For this review, take the finished solid that the model builds, in its own axes (mm). A direction names the side the tool comes from. Coordinates: 2 decimals unless noted, no trailing zeros. Loops run counter-clockwise (first coordinate to the right, second up) from the corner with the lowest first, then second, coordinate; pieces in that order, holes last. Notation, with made-up numbers: M 15,67 L 65,67 A26 ccw 65,85 Z; hole C 69.25,-18 d8. An arc over 180 degrees is marked long. Answer as a JSON object with one key per item and string values. Group by question number.
Item 1: Add section B-B (z = -44). State the section outline as (x, y) points, then the cut area to 3 significant figures.
Item 2: Add section D-D (y = 3.5). State the section outline as (x, z) points.
Item 3: Add section A-A (y = 22). State the section outline as (x, z) points, then the cut area to 3 significant figures.
Item 4: Insertion check: pin 1 (6 mm diameter, centred on x = -32, y = 5.5, fed in from -Z); pin 2 (6 mm diameter, centred on x = -5.5, z = -49.5, fed in from +Y); pin 3 (5 mm diameter, centred on x = -46.5, y = 19.5, fed in from -Z). Each pin has a flat end and moves straight along its axis. Give the tip position at first contact, or say it passes through.
Item 5: Wall thickness on L1, parallel to Z at x = -88.5, y = 27; L2, parallel to Y at x = 7, z = -45; L3, parallel to X at y = 8, z = -52: over which ranges is each line inside the solid? List them lowest first. Write a range as from..to.
Item 6: Tool access review of faces 5 (the face through (-41, 23, -42.5)), 6 (the face through (7, 2.5, -49)), 7 (the face through (-41, 30.911, -37)): name each direction out of +Z, -Z, +X, -X, +Y, -Y from which nothing blocks a thin tool from reaching the whole face with its end or side.
Item 7: Mouldability with a two-part tool opening along Z and no side actions: class faces 1 (the face through (-81, 15, -47)), 2 (the face through (-41, 16, -32.5)), 3 (the face through (7.057, 8.838, -51.855)), 4 (the face through (-40.9, 7.4, -42.5)) as +Z half, -Z half, draft (parallel to the pull), parting line (faces both ways), or undercut.
Item 8: Add section C-C (x = -61.5). State the section outline as (y, z) points, then the cut area to 3 significant figures.
from build123d import *

# Parameters (mm, degrees)
BOSS_EXTRUDE1_DEPTH = 15
SKETCH5_W           = 107
SKETCH5_H           = 15.91087052
BOSS_EXTRUDE2_DEPTH = 10
CUT_EXTRUDE1_START  = -15
SKETCH6_R           = 2.9
CUT_EXTRUDE1_DEPTH  = 12.5
SKETCH7_R           = 2.9
CUT_EXTRUDE2_DEPTH  = 12.5


with BuildPart() as part:
    # Sketch4 → Boss-Extrude1 (new body)
    with BuildSketch(Plane(origin=(0, 0, 0), x_dir=(1, 0, 0), z_dir=(0, 1, 0))):
        with BuildLine():
            Line((13.184906132, 32.500351338), (-93.815093868, 32.500351338))
            Line((-93.815093868, 32.500351338), (-93.815093868, 48.957491145))
            ThreePointArc((-93.815093868, 48.957491145), (-87.815093868, 54.957491145), (-81.815093868, 48.957491145))
            ThreePointArc((-81.815093868, 48.957491145), (-40.315093868, 42.500341518), (1.184906132, 48.957491145))
            ThreePointArc((1.184906132, 48.957491145), (7.184906132, 54.957491145), (13.184906132, 48.957491145))
            Line((13.184906132, 48.957491145), (13.184906132, 32.500351338))
        make_face()
    extrude(amount=BOSS_EXTRUDE1_DEPTH)

    # Sketch5 → Boss-Extrude2 (add)
    with BuildSketch(Plane.XY.offset(-32.500351338)):
        with Locations((-40.315093868, 22.95543526)):
            Rectangle(SKETCH5_W, SKETCH5_H)
    extrude(amount=-BOSS_EXTRUDE2_DEPTH)

    # Sketch6 → Cut-Extrude1 (cut)
    with BuildSketch(Plane.XZ.offset(CUT_EXTRUDE1_START)):
        with Locations(Location((7.184906132, -48.957491145, 0), (0, 0, 90))):
            Circle(SKETCH6_R)
        with Locations(Location((-87.815093868, -48.957491145, 0), (0, 0, 90))):
            Circle(SKETCH6_R)
    extrude(amount=CUT_EXTRUDE1_DEPTH, mode=Mode.SUBTRACT)

    # Sketch7 → Cut-Extrude2 (cut)
    with BuildSketch(Plane(origin=(0, 0, -42.500351338), x_dir=(-1, 0, 0), z_dir=(0, 0, -1))):
        with Locations((-7.184906132, 22)):
            Circle(SKETCH7_R)
        with Locations((87.815093868, 22)):
            Circle(SKETCH7_R)
    extrude(amount=-CUT_EXTRUDE2_DEPTH, mode=Mode.SUBTRACT)


solid = part.part
From the geometry:
{
 "1": {"outline": "M -93.82,0 L -60.5,0 L -60.5,15 L -93.82,15 Z; M -20.13,0 L 13.18,0 L 13.18,15 L -20.13,15 Z", "area": "999 mm²"},
 "2": {"outline": "M -93.82,-48.96 A6 ccw -81.82,-48.96 A136.59 cw 1.18,-48.96 A6 ccw 13.18,-48.96 L 13.18,-32.5 L -93.82,-32.5 Z; hole C -87.82,-48.96 d5.8; hole C 7.18,-48.96 d5.8"},
 "3": {"outline": "M -93.82,-42.5 L -90.72,-42.5 L -90.72,-32.5 L -93.82,-32.5 Z; M -84.92,-42.5 L 4.28,-42.5 L 4.28,-32.5 L -84.92,-32.5 Z; M 10.08,-42.5 L 13.18,-42.5 L 13.18,-32.5 L 10.08,-32.5 Z", "area": "954 mm²"},
 "4": {"pin 1": "stops at z = -42.97", "pin 2": "stops at y = 15", "pin 3": "stops at z = -42.5"},
 "5": {"L1": "z = -42.5..-32.5", "L2": "y = 0..15", "L3": "x = -92.99..-82.64, 2.01..12.36"},
 "6": {"face 5": "-Z, +X, -X, +Y", "face 6": "+Y", "face 7": "+Z, -Z, +X, -X, +Y"},
 "7": {"face 1": "draft", "face 2": "+Z half", "face 3": "undercut", "face 4": "-Z half"},
 "8": {"outline": "M 0,-44.15 L 15,-44.15 L 15,-42.5 L 30.91,-42.5 L 30.91,-32.5 L 0,-32.5 Z", "area": "334 mm²"}
}
